Can you work these out from the drawing? Everything is in mm from the part's minimum corner. Round coordinates to 2 decimals unless told otherwise and drop trailing zeros. Loops run counter-clockwise (first coordinate to the right, second up) from the corner with the lowest first, then second, coordinate; pieces in that order, holes last. Notation, with made-up numbers: (3.5, -25.5) -> (34.5, -25.5) arc R19 ccw to (34.5, -3.5) -> close; hole circle Ø10 at (58, -33). An arc over 180 degrees is marked (long way). Use CSV: the item, a comma, the result in double quotes. Start each with the question number.
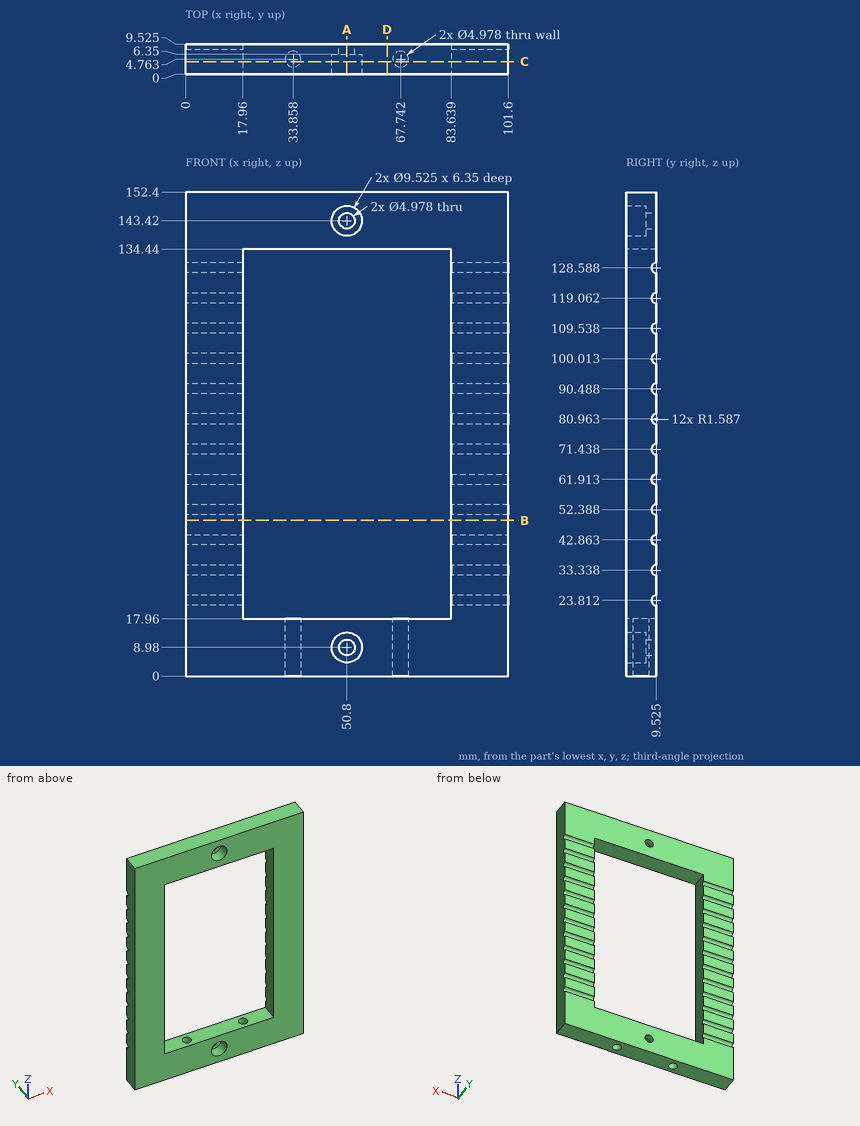
1. Suppose I cut it at C-C (y = 4). List the corners of the cut face in (x, z) for me (1 decimal).
2. Will these pins go through, and if not, where does the flat tip stop? pin 1 (3 mm diameter, centred on x = 49.5, z = 9, fed in from -Y); pin 2 (3 mm diameter, centred on x = 67.74, y = 4.76, fed in from -Z); pin 3 (15 mm diameter, centred on x = 50.8, z = 8.98, fed in from -Y); pin 4 (4.5 mm diameter, centred on x = 50.8, z = 8.98, fed in from -Y).
3. Suppose I cut it at A-A (x = 50.8). State how many separate pieces and enclosed holes the cut face has.
4. Suppose I cut it at B-B (z = 49). List the corners of the cut face in (x, y) for me (1 decimal), then the cut area to 3 significant figures.
5. If I drill on L1, parallel to Z at x = 50.8, y = 4.75; L2, parallel to Z at x = 50.8, y = 8.4; L3, parallel to X at y = 6, z = 83.5, over which ranges is the centre line in solid material (lowest first)?
6. Suppose I cut it at D-D (x = 63.5). List the corners of the cut face in (y, z) for me (1 decimal).
Geometry check:
1,outline,"(0, 0) -> (31.5, 0) -> (31.5, 18) -> (18, 18) -> (18, 134.4) -> (83.6, 134.4) -> (83.6, 18) -> (70.1, 18) -> (70.1, 0) -> (101.6, 0) -> (101.6, 152.4) -> (0, 152.4) -> close; (36.2, 0) -> (65.4, 0) -> (65.4, 18) -> (36.2, 18) -> close; hole circle Ø9.5 at (50.8, 9); hole circle Ø9.5 at (50.8, 143.4)"
2,pin 1,"stops at y = 6.35"
2,pin 2,"stops at z = 134.44"
2,pin 3,"stops at y = 0"
2,pin 4,"passes through"
3,separate pieces,"4"
3,enclosed holes,"0"
4,outline,"(0, 0) -> (18, 0) -> (18, 9.5) -> (0, 9.5) -> close; (83.6, 0) -> (101.6, 0) -> (101.6, 9.5) -> (83.6, 9.5) -> close"
4,area,"342 mm²"
5,L1,"z = 0 to 4.22, 13.74 to 17.96, 134.44 to 138.66, 148.18 to 152.4"
5,L2,"z = 0 to 6.49, 11.47 to 17.96, 134.44 to 140.93, 145.91 to 152.4"
5,L3,"x = 0 to 17.96, 83.64 to 101.6"
6,outline,"(0, 0) -> (9.5, 0) -> (9.5, 18) -> (0, 18) -> close; (0, 134.4) -> (9.5, 134.4) -> (9.5, 152.4) -> (0, 152.4) -> close"
